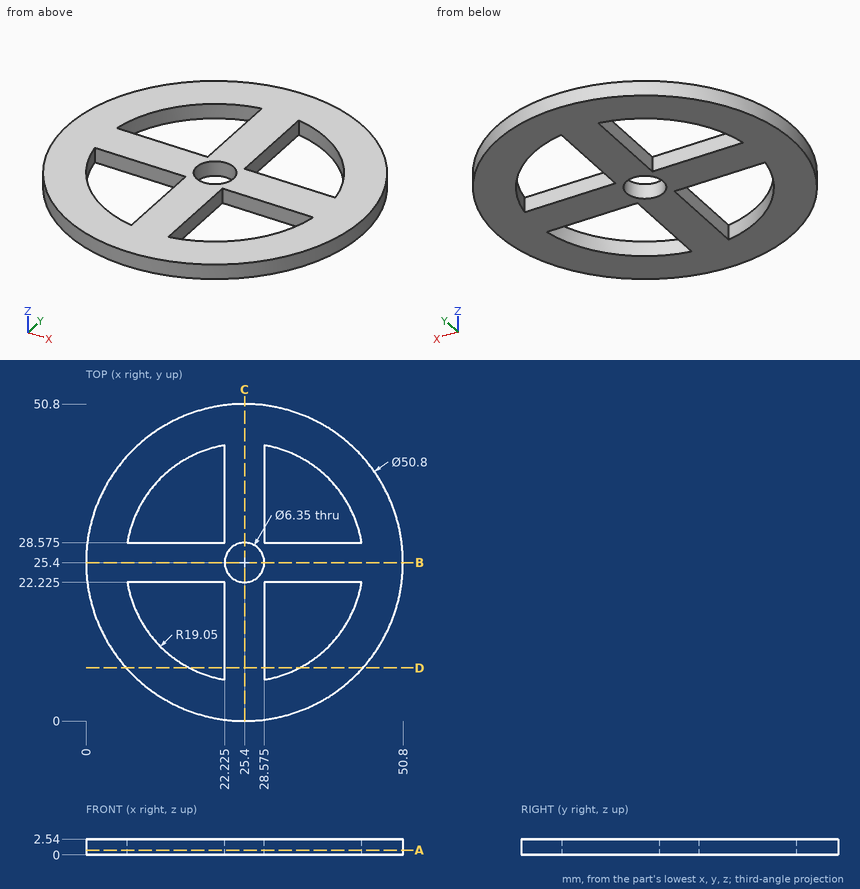
Here's the drawing with two shaded views (mm, measured from the low corner). I have some questions. Coordinates: 2 decimals unless noted, no trailing zeros. Loops run counter-clockwise (first coordinate to the right, second up) from the corner with the lowest first, then second, coordinate; pieces in that order, holes last. Notation, with made-up numbers: M -10,13 L 29,13 A24 cw 29,31 Z; hole C 60.5,28 d11. An arc over 180 degrees is marked long. Return JSON: item names as keys, results as strings. Group by question number.
Item 1: I'm going to push flat-ended pins straight in: pin 1 Ø4 at (x, y) = (25.4, 25.4) entering from -Z; pin 2 Ø0.8 at (y, z) = (33.5, 2) entering from +X; pin 3 Ø1.3 at (y, z) = (37, 1.5) entering from -X. Where does each tip first touch, or does it pass through?
Item 2: Imagine slicing it at B-B (y = 25.4). Please give me the cut outline in (x, z) (3 decimals), and give its area (3 significant figures).
Item 3: If I drill on L1, parallel to X at y = 22, z = 1.1 (3 decimals); L2, parallel to Y at x = 13.5, z = 0.85 (3 decimals); L3, parallel to Y at x = 25.4, z = 0.8 (3 decimals), over which ranges is the centre line in solid material (lowest first)? Write a range as from..to.
Item 4: Imagine slicing it at A-A (z = 0.75). Please give me the cut outline in (x, y) (3 decimals), and give its area (3 significant figures).
Item 5: Imagine slicing it at D-D (y = 8.5). Please give me the cut outline in (x, z) (3 decimals), and give its area (3 significant figures).
Verdict:
{
 "1": {"pin 1": "passes through", "pin 2": "stops at x = 49.6", "pin 3": "stops at x = 2.48"},
 "2": {"outline": "M 0,0 L 22.225,0 L 22.225,2.54 L 0,2.54 Z; M 28.575,0 L 50.8,0 L 50.8,2.54 L 28.575,2.54 Z", "area": "113 mm^2"},
 "3": {"L1": "x = 0.229..6.656, 22.225..28.575, 44.144..50.571", "L2": "y = 2.96..10.524, 22.225..28.575, 40.276..47.84", "L3": "y = 0..22.225, 28.575..50.8"},
 "4": {"outline": "C 25.4,25.4 d50.8; hole M 6.616,22.225 A19.05 ccw 22.225,6.616 L 22.225,22.225 Z; hole M 6.616,28.575 L 22.225,28.575 L 22.225,44.184 A19.05 ccw Z; hole C 25.4,25.4 d6.35; hole M 28.575,6.616 A19.05 ccw 44.184,22.225 L 28.575,22.225 Z; hole M 28.575,28.575 L 44.184,28.575 A19.05 ccw 28.575,44.184 Z", "area": "1,300 mm^2"},
 "5": {"outline": "M 6.438,0 L 16.608,0 L 16.608,2.54 L 6.438,2.54 Z; M 22.225,0 L 28.575,0 L 28.575,2.54 L 22.225,2.54 Z; M 34.192,0 L 44.362,0 L 44.362,2.54 L 34.192,2.54 Z", "area": "67.8 mm^2"}
}
